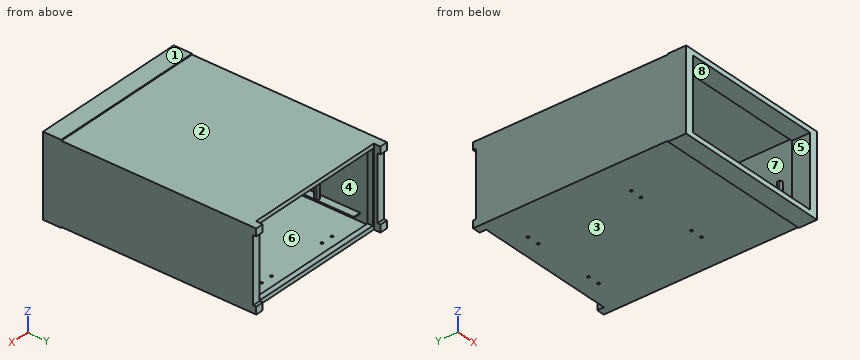
```python
from build123d import *

# Parameters (mm, degrees)
F0_W      = 260
F0_H      = 350
F1_DEPTH  = 133
F2_W      = 260
F2_H      = 330
F3_DEPTH  = 1.5
F4_W      = 260
F4_H      = 330
F5_DEPTH  = 1.5
F6_W      = 234
F6_H      = 11
F7_DEPTH  = 131.501
F10_R     = 2
F11_DEPTH = 25
F12_W     = 239
F12_H     = 128
F13_DEPTH = 330.5
F14_W     = 260
F14_H     = 133
F14_W_2   = 233
F14_H_2   = 116.5
F15_DEPTH = 30
F9_W      = 13
F9_H      = 106
F8_W      = 13
F8_H      = 106
F16_DEPTH = 5
F17_W     = 230
F17_H     = 116.25
F18_DEPTH = 25
F19_W     = 281.5
F19_H     = 1.6
F20_DEPTH = 12.5
F21_W     = 281.5
F21_H     = 1.6
F22_DEPTH = 12.5
F23_R     = 2
F24_DEPTH = 50


with BuildPart() as f1:
    # F0 (on Top) → F1 (new body)
    with BuildSketch(Plane.XY):
        Rectangle(F0_W, F0_H)
    extrude(amount=F1_DEPTH)

    # F2 (on face) → F3 (cut)
    with BuildSketch(Plane.XY.offset(133)):
        with Locations((0, 10)):
            Rectangle(F2_W, F2_H)
    extrude(amount=-F3_DEPTH, mode=Mode.SUBTRACT)

    # F4 (on face) → F5 (cut)
    with BuildSketch(Plane(origin=(0, 0, 0), x_dir=(1, 0, 0), z_dir=(0, 0, -1))):
        with Locations((0, -10)):
            Rectangle(F4_W, F4_H)
    extrude(amount=-F5_DEPTH, mode=Mode.SUBTRACT)

    # F6 (on face) → F7 (cut, through all)
    with BuildSketch(Plane.XY.offset(131.5)):
        with Locations((0, 169.5)):
            Rectangle(F6_W, F6_H)
    extrude(amount=-F7_DEPTH, mode=Mode.SUBTRACT)

    # F10 (on face) → F11 (cut)
    with BuildSketch(Plane(origin=(0, 0, 1.5), x_dir=(1, 0, 0), z_dir=(0, 0, -1))):
        with Locations((70, 35)):
            Circle(F10_R)
        with Locations((50, 35)):
            Circle(F10_R)
        with Locations((-70, 35)):
            Circle(F10_R)
        with Locations((-50, 35)):
            Circle(F10_R)
        with Locations((70, -134)):
            Circle(F10_R)
        with Locations((50, -134)):
            Circle(F10_R)
        with Locations((-50, -134)):
            Circle(F10_R)
        with Locations((-70, -134)):
            Circle(F10_R)
    extrude(amount=-F11_DEPTH, mode=Mode.SUBTRACT)

    # F12 (on face) → F13 (cut)
    with BuildSketch(Plane.XZ.offset(175)):
        with Locations((0, 66.5)):
            Rectangle(F12_W, F12_H)
    extrude(amount=-F13_DEPTH, mode=Mode.SUBTRACT)

    # F14 (on face) → F15 (join)
    with BuildSketch(Plane.XZ.offset(175)):
        with Locations((0, 66.5)):
            Rectangle(F14_W, F14_H)
        with Locations((0, 66.5)):
            Rectangle(F14_W_2, F14_H_2, mode=Mode.SUBTRACT)
    extrude(amount=-F15_DEPTH)

    # F9 (on face) + F8 (on face) → F16 (cut)
    with BuildSketch(Plane(origin=(0, 175, 0), x_dir=(-1, 0, 0), z_dir=(0, 1, 0))):
        with Locations((-123.5, 66.5)):
            Rectangle(F9_W, F9_H)
    with BuildSketch(Plane(origin=(0, 175, 0), x_dir=(-1, 0, 0), z_dir=(0, 1, 0))):
        with Locations((123.5, 66.5)):
            Rectangle(F8_W, F8_H)
    extrude(amount=-F16_DEPTH, mode=Mode.SUBTRACT)

    # F17 (on face) → F18 (cut)
    with BuildSketch(Plane(origin=(0, 175, 0), x_dir=(-1, 0, 0), z_dir=(0, 1, 0))):
        with Locations((0, 66.5)):
            Rectangle(F17_W, F17_H)
    extrude(amount=-F18_DEPTH, mode=Mode.SUBTRACT)

    # F19 (on face) → F20 (join)
    with BuildSketch(Plane.YZ.offset(-119.5)):
        with Locations((-1.25, 14.8)):
            Rectangle(F19_W, F19_H)
    extrude(amount=F20_DEPTH)

    # F21 (on face) → F22 (join)
    with BuildSketch(Plane(origin=(119.5, 0, 0), x_dir=(0, -1, 0), z_dir=(-1, 0, 0))):
        with Locations((1.25, 14.8)):
            Rectangle(F21_W, F21_H)
    extrude(amount=F22_DEPTH)

    # F23 (on face) → F24 (join)
    with BuildSketch(Plane.XY.offset(15.6)):
        Polygon((111, -134.041452), (114.5, -132.020726), (114.5, -127.979274), (111, -125.958548), (107.5, -127.979274), (107.5, -132.020726), align=None)
        with Locations((111, -130)):
            Circle(F23_R, mode=Mode.SUBTRACT)
        Polygon((111, 71.958548), (114.5, 73.979274), (114.5, 78.020726), (111, 80.041452), (107.5, 78.020726), (107.5, 73.979274), align=None)
        with Locations((111, 76)):
            Circle(F23_R, mode=Mode.SUBTRACT)
        Polygon((111, -31.041452), (114.5, -29.020726), (114.5, -24.979274), (111, -22.958548), (107.5, -24.979274), (107.5, -29.020726), align=None)
        with Locations((111, -27)):
            Circle(F23_R, mode=Mode.SUBTRACT)
        Polygon((-111, -134.041452), (-107.5, -132.020726), (-107.5, -127.979274), (-111, -125.958548), (-114.5, -127.979274), (-114.5, -132.020726), align=None)
        with Locations((-111, -130)):
            Circle(F23_R, mode=Mode.SUBTRACT)
        Polygon((-107.5, -29.020726), (-107.5, -24.979274), (-111, -22.958548), (-114.5, -24.979274), (-114.5, -29.020726), (-111, -31.041452), align=None)
        with Locations((-111, -27)):
            Circle(F23_R, mode=Mode.SUBTRACT)
        Polygon((-111, 71.958548), (-107.5, 73.979274), (-107.5, 78.020726), (-111, 80.041452), (-114.5, 78.020726), (-114.5, 73.979274), align=None)
        with Locations((-111, 76)):
            Circle(F23_R, mode=Mode.SUBTRACT)
    extrude(amount=F24_DEPTH)


solid = f1.part
```
Work out the finished part from the listing and answer in its coordinate system (mm). Face numbers are marked on the shaded views. A direction names the side the tool comes from. Give positions to 0.01 mm unless a question says otherwise; leave off trailing zeros. Loops run counter-clockwise (first coordinate to the right, second up) from the corner with the lowest first, then second, coordinate; pieces in that order, holes last. Notation, with made-up numbers: (85, 1.5) - (96, 1.5) arc R19 ccw to (96, 37.5) - close; hole circle Ø10 at (2, -0.75). An arc over 180 degrees is marked (long way). Use CSV: the item, a comma, the result in double quotes. Start each with the question number.
(1) Find the intervals of material crossed by L1, parallel to Y at x = -111, z = 42; L2, parallel to Y at x = -50, z = 2.25; L3, parallel to X at y = 134, z = 1.8, in increasing order.
(2) Determine the mould class of the marked faces 6, 7 and 8 for opening direction Y: released by +Y, released by -Y, zero draft, split by the parting line, or undercut.
(3) Find section D-D, the plane z = 57. Count the separate pieces of the cut face and the enclosed holes in it, plus the area to 3 significant figures.
(4) Find section C-C, the plane y = -67. Determine the outline of the cut face in (x, z), plus the area to 3 significant figures.
(5) Find section B-B, the plane x = 77. Determine the outline of the cut face in (y, z) (3 decimals).
(6) A tool of negligible diameter and unlimited length cuts with its end or side. For the marked faces 1, 2, 3, 4 and 5, from which of +Z, -Z, +X, -X, +Y, -Y can it reach the whole face along a straight path? Write none if from no direction.
(7) Each of these flat-tipped pins is pushed along its axis until it touches: pin 1 (10 mm diameter, centred on x = -39, y = 68, fed in from -Z); pin 2 (1.6 mm diameter, centred on x = 5.5, z = 132, fed in from +Y); pin 3 (2.5 mm diameter, centred on x = -70, y = 134, fed in from -Z). Where does it stop, or does it pass through?
(8) Find section A-A, the plane z = 91. Determine the outline of the cut face in (x, y).
Results found:
1,L1,"-134.04 to -132, -128 to -125.96, -31.04 to -29, -25 to -22.96, 71.96 to 74, 78 to 80.04"
1,L2,"-175 to -37, -33 to 132, 136 to 164"
1,L3,"-130 to -72, -68 to -52, -48 to 48, 52 to 68, 72 to 130"
2,face 6,"undercut"
2,face 7,"undercut"
2,face 8,"zero draft"
3,separate pieces,"8"
3,enclosed holes,"6"
3,area,"7,710 mm^2"
4,outline,"(-130, 1.5) - (130, 1.5) - (130, 131.5) - (-130, 131.5) - close; hole (-119.5, 2.5) - (119.5, 2.5) - (119.5, 14) - (107, 14) - (107, 15.6) - (119.5, 15.6) - (119.5, 130.5) - (-119.5, 130.5) - (-119.5, 15.6) - (-107, 15.6) - (-107, 14) - (-119.5, 14) - close"
4,area,"3,250 mm^2"
5,outline,"(-175, 0) - (-145, 0) - (-145, 1.5) - (164, 1.5) - (164, 8.375) - (155.5, 8.375) - (155.5, 2.5) - (-145, 2.5) - (-145, 8.25) - (-175, 8.25) - close; (-175, 124.75) - (-145, 124.75) - (-145, 130.5) - (155.5, 130.5) - (155.5, 124.625) - (164, 124.625) - (164, 131.5) - (-145, 131.5) - (-145, 133) - (-175, 133) - close"
6,face 1,"+Z, +X, -X, +Y, -Y"
6,face 2,"+Z, +X, -X, +Y"
6,face 3,"-Z, +X, -X, +Y"
6,face 4,"none"
6,face 5,"-Y"
7,pin 1,"z = 1.5"
7,pin 2,"y = 164"
7,pin 3,"z = 130.5"
8,outline,"(-130, -175) - (-116.5, -175) - (-116.5, -145) - (-119.5, -145) - (-119.5, 155.5) - (-115, 155.5) - (-115, 164) - (-117, 164) - (-117, 170) - (-130, 170) - close; (115, 155.5) - (119.5, 155.5) - (119.5, -145) - (116.5, -145) - (116.5, -175) - (130, -175) - (130, 170) - (117, 170) - (117, 164) - (115, 164) - close"
